Geometry: final body of the model. Coordinates: model frame, mm. A direction names the side the tool comes from. Coordinates: 2 decimals unless noted, no trailing zeros.
Autodesk Inventor part; units mm, degrees
ref_plane "YZ Plane" through (0, 0, 0) normal (1, 0, 0) x (0, 1, 0)
ref_plane "XZ Plane" through (0, 0, 0) normal (0, 1, 0) x (-1, 0, 0)
ref_plane "XY Plane" through (0, 0, 0) normal (0, 0, 1) x (1, 0, 0)
ref_plane "Work Plane1" through (0, 0, 0) normal (0, 0, 1) x (1, 0, 0)
sketch "Sketch1" plane through (0, 0, 0) normal (0, 0, 1) x (1, 0, 0)
  circle A0 centre (-21, 106) radius 1.45
  circle A1 centre (-21, 69.5) radius 1.45
  circle A2 centre (-21, 33) radius 1.45
  circle A3 centre (-21, -3.5) radius 1.45
  circle A4 centre (-21, -40) radius 1.45
  circle A5 centre (-21, -113) radius 1.45
  circle A6 centre (21, -113) radius 1.45
  circle A7 centre (21, -40) radius 1.45
  circle A8 centre (21, -3.5) radius 1.45
  circle A9 centre (21, 33) radius 1.45
  circle A10 centre (21, 69.5) radius 1.45
  circle A11 centre (21, 106) radius 1.45
  arc A12 (-6.5, 102) -> (-11.5, 97) centre (-6.5, 97) ccw
  line L0 (-6.5, 102) -> (6.5, 102)
  arc A13 (11.5, 97) -> (6.5, 102) centre (6.5, 97) ccw
  line L1 (11.5, 97) -> (11.5, -97)
  arc A14 (6.5, -102) -> (11.5, -97) centre (6.5, -97) ccw
  line L2 (6.5, -102) -> (-6.5, -102)
  arc A15 (-11.5, -97) -> (-6.5, -102) centre (-6.5, -97) ccw
  line L3 (-11.5, -97) -> (-11.5, 97)
  arc A16 (25.5, -118) -> (27.5, -116) centre (25.5, -116) ccw
  line L4 (27.5, -116) -> (27.5, 116)
  arc A17 (27.5, 116) -> (25.5, 118) centre (25.5, 116) ccw
  line L5 (25.5, 118) -> (-25.5, 118)
  arc A18 (-25.5, 118) -> (-27.5, 116) centre (-25.5, 116) ccw
  line L6 (-27.5, 116) -> (-27.5, -116)
  arc A19 (-27.5, -116) -> (-25.5, -118) centre (-25.5, -116) ccw
  line L7 (-25.5, -118) -> (25.5, -118)
  circle A20 centre (21, -76.5) radius 1.45
  circle A21 centre (-21, -76.5) radius 1.45
  circle A22 centre (21, 111.5) radius 1.45
  circle A23 centre (-21, 111.5) radius 1.45
  arc A24 (48.8107, 3.6492) -> (48.6958, 3.3718) centre (50.5958, 2.7473) ccw construction
  line L8 (48.6958, -66.1718) -> (48.6958, 3.3718) construction
  arc A25 (48.6958, -66.1718) -> (48.8107, -66.4492) centre (50.5958, -65.5473) ccw construction
  line L9 (54.3466, -71.9851) -> (48.8107, -66.4492) construction
  arc A26 (54.3466, -71.9851) -> (54.624, -72.1) centre (55.2485, -70.2) ccw construction
  line L10 (170.6958, -72.1) -> (54.624, -72.1) construction
  arc A27 (170.6958, -72.1) -> (172.2958, -70.5) centre (170.6958, -70.5) ccw construction
  line L11 (172.2958, 7.7) -> (172.2958, -70.5) construction
  arc A28 (172.2958, 7.7) -> (170.6958, 9.3) centre (170.6958, 7.7) ccw construction
  line L12 (54.624, 9.3) -> (170.6958, 9.3) construction
  arc A29 (54.624, 9.3) -> (54.3466, 9.1851) centre (55.2485, 7.4) ccw construction
  line L13 (48.8107, 3.6492) -> (54.3466, 9.1851) construction
  line L14 (56.1958, 4.9) -> (164.7958, 4.9) construction
  line L15 (164.7958, 4.9) -> (164.7958, -67.7) construction
  line L16 (164.7958, -67.7) -> (56.1958, -67.7) construction
  line L17 (56.1958, -67.7) -> (56.1958, 4.9) construction
  line L18 (174.3958, -70.2) -> (174.3958, 7.4) construction
  arc A30 (50.5958, 11.1) -> (46.8958, 7.4) centre (50.5958, 7.4) ccw construction
  arc A31 (46.6958, -70.2) -> (50.5958, -74.1) centre (50.5958, -70.2) ccw construction
  arc A32 (174.2958, 7.4) -> (170.3958, 11.3) centre (170.3958, 7.4) ccw construction
  arc A33 (170.3958, -74.1) -> (174.2958, -70.2) centre (170.3958, -70.2) ccw construction
  line L19 (-27.5, -118) -> (182.5, -118)
  line L20 (182.5, -118) -> (182.5, -102)
  line L21 (182.5, -102) -> (-27.5, -102)
  line L22 (-27.5, -102) -> (-27.5, -118)
  circle A34 centre (21, -113) radius 1.45 construction
  circle A35 centre (-21, -113) radius 1.45 construction
  line L23 (27.5, -102) -> (11.5, -102)
  line L24 (11.5, -102) -> (11.5, -70)
  line L25 (11.5, -70) -> (27.5, -70)
  line L26 (27.5, -70) -> (27.5, -102)
  line L27 (-27.5, -102) -> (-11.5, -102)
  line L28 (-11.5, -102) -> (-11.5, -70)
  line L29 (-11.5, -70) -> (-27.5, -70)
  line L30 (-27.5, -70) -> (-27.5, -102)
  circle A36 centre (21, -76.5) radius 1.45
  circle A37 centre (-21, -76.5) radius 1.45
  circle A38 centre (21, -113) radius 1.45
  circle A39 centre (-21, -113) radius 1.45
  circle A40 centre (21, -113) radius 1.45
  circle A41 centre (-21, -113) radius 1.45
  circle A42 centre (15.5, -113) radius 1.45
  circle A43 centre (57.5, -113) radius 1.45
  circle A44 centre (52, -113) radius 1.45
  circle A45 centre (94, -113) radius 1.45
  circle A46 centre (88.5, -113) radius 1.45
  circle A47 centre (130.5, -113) radius 1.45
  circle A48 centre (125, -113) radius 1.45
  circle A49 centre (167, -113) radius 1.45
  circle A50 centre (161.5, -113) radius 1.45
  circle A51 centre (203.5, -113) radius 1.45
  circle A52 centre (198, -113) radius 1.45
  circle A53 centre (240, -113) radius 1.45
  circle A54 centre (234.5, -113) radius 1.45
  circle A55 centre (276.5, -113) radius 1.45
  circle A56 centre (271, -113) radius 1.45
  circle A57 centre (313, -113) radius 1.45
  circle A58 centre (307.5, -113) radius 1.45
  circle A59 centre (349.5, -113) radius 1.45
  point P0 (0, 0)
  dimension "d1" = 210
  dimension "d2" = 32
  dimension "d8" = 36.5
extrude "Extrusion1" add sketch "Sketch1" along normal blind 6 contours L2 L21 L4 A16 L7 A19 L6 | A19 L19 L22 | L21 L20 L19 A16 L4 | A42 | A43 | A44 | A45 | A46 | A47 | A48 | A49 | A50
fillet "Fillet1" radius 2 2 edges at (-27.5, -118, 3) (182.5, -118, 3)
sketch "Sketch2" plane through (0, 0, 6) normal (0, 0, 1) x (1, 0, 0)
  arc A0 (180.5, -118) -> (182.5, -116) centre (180.5, -116) ccw
  line L0 (182.5, -116) -> (182.5, -102)
  line L1 (182.5, -102) -> (-27.5, -102)
  line L2 (-27.5, -102) -> (-27.5, -116)
  arc A1 (-27.5, -116) -> (-25.5, -118) centre (-25.5, -116) ccw
  line L3 (-25.5, -118) -> (180.5, -118)
  line L4 (-25.1, -118) -> (-25.1, -108)
  point P0 (0, 0)
  point P1 (57.5, -113)
  point P2 (15.5, -113)
  point P3 (94, -113)
  point P4 (52, -113)
  point P5 (130.5, -113)
  point P6 (88.5, -113)
  point P7 (167, -113)
  point P8 (125, -113)
  point P9 (203.5, -113)
  point P10 (161.5, -113)
  point P11 (240, -113)
  point P12 (198, -113)
  point P13 (276.5, -113)
  point P14 (234.5, -113)
  point P15 (313, -113)
  point P16 (271, -113)
  point P17 (349.5, -113)
  point P18 (307.5, -113)
  dimension "d15" = 36.5
hole "Hole1" at (15.5, -113, 6) at (52, -113, 6) at (57.5, -113, 6) at (88.5, -113, 6) at (94, -113, 6) at (125, -113, 6) at (130.5, -113, 6) at (161.5, -113, 6) at (167, -113, 6) direction (0, 0, -1) diameter 2.9 end through all counterbore diameter 6.5 counterbore depth 3
properties part number "03_Opentrons_Microscope_MTP_stand"
Item 1: Pull-direction query (Y, two-part tool) for faces 1 (the cylindrical face through (85.252, -113.117, 4.479)), 2 (the flat face through (79, -102, 3)), 3 (the flat face through (76, -110, 0)); classes: released by +Y, released by -Y, zero draft, split by the parting line, or undercut.
Derived:
face 1: undercut
face 2: released by +Y
face 3: zero draft
Item 2: Section A-A, the plane z = 1.7. State how many separate pieces and enclosed holes the cut face has, plus the area to 3 significant figures.
Derived:
separate pieces: 1
enclosed holes: 11
area: 3,290 mm2
Item 3: Set-up query: faces 4 (the flat face through (55, -113, 3)), 5 (the flat face through (182.5, -109, 3)). Return all of +Z, -Z, +X, -X, +Y, -Y with unobstructed straight access to the full face (end or side cutting, diameter ignored); none if empty.
Derived:
face 4: +Z
face 5: +Z, -Z, +X, +Y, -Y
Item 4: Pin query (flat end, axial travel): pin 1 (2.5 mm diameter, centred on x = 15.5, y = -113, fed in from -Z); pin 2 (4 mm diameter, centred on x = 88.5, y = -113, fed in from +Z). Return the tip coordinate at first contact, or that it passes through.
Derived:
pin 1: passes through
pin 2: stops at z = 3
Item 5: Material intervals for probe 1 along Y at (x, z) = (167, 4.2); probe 2 along Y at (x, z) = (57.5, 1.65); probe 3 along Z at (x, y) = (52, -110), sorted ascending.
Derived:
probe 1: y = -118 to -116.25, -109.75 to -102
probe 2: y = -118 to -114.45, -111.55 to -102
probe 3: z = 0 to 3
